```python
from build123d import *

# Parameters (mm, degrees)
SKETCH1_W      = 38.1
SKETCH1_H      = 38.1
BASEHEAD_DEPTH = 17.3736


with BuildPart() as part:
    # Sketch1 → BaseHead (new body)
    with BuildSketch(Plane(origin=(0, 0, 0), x_dir=(0, 0.7071067811865488, -0.7071067811865462), z_dir=(1, 0, 0))):
        Rectangle(SKETCH1_W, SKETCH1_H)
    extrude(amount=BASEHEAD_DEPTH)

    # BodySke → Body (revolve)
    with BuildSketch(Plane.XY, mode=Mode.PRIVATE) as body_sk:
        Polygon((17.3736, 0), (17.3736, 12.7), (91.6813, 12.7), (93.5736, 10.8077), (93.5736, 0), align=None)
    revolve(body_sk.sketch.rotate(Axis((0, 0, 0), (1, 0, 0)), 90), axis=Axis((0, 0, 0), (1, 0, 0)))

    # Sketch3 → HeadChamfer (revolve, cut)
    with BuildSketch(Plane.XY):
        Polygon((0, 19.05), (-12.7, 19.05), (-12.7, 52.340768363), (15.523740234, 52.340768363), align=None)
    revolve(axis=Axis((0, 0, 0), (1, 0, 0)), mode=Mode.SUBTRACT)


solid = part.part
```
Here's how the part is built. I have some questions about the finished solid (model axes, mm). A direction names the side the tool comes from. Give positions to 0.01 mm unless a question says otherwise; leave off trailing zeros. Loops run counter-clockwise (first coordinate to the right, second up) from the corner with the lowest first, then second, coordinate; pieces in that order, holes last. Notation, with made-up numbers: M -24.75,36.25 L 20.25,36.25 A24 cw 20.25,56.25 Z; hole C 14.25,-15.5 d11. An arc over 180 degrees is marked long. Put each result on its own line as item: value. Start each with the question number.
(1) I want a section at B-B on x = 30. Please give me the cut outline in (y, z), then the cut area to 3 significant figures.
(2) Will these pins go through, and if not, where does the flat tip stop? pin 1 Ø6 at (y, z) = (5.5, -13) entering from +X; pin 2 Ø1 at (y, z) = (3.5, 1) entering from -X; pin 3 Ø1 at (x, z) = (81.5, 11) entering from +Y; pin 4 Ø1.5 at (x, z) = (27.5, -6) entering from -Y.
(3) I want a section at A-A on x = 11.5. Please give me the cut outline in (y, z), then the cut area to 3 significant figures.
(4) If we mould it in two halves opening along X, with no side actions, what happens to faces 3 (the flat face through (0, 0, 0)), 4 (the flat face through (93.574, 0, 0)), 5 (the flat face through (8.57, -13.66, -13.28))? For each: +X half, -X half, draft (parallel to the pull), parting line (faces both ways), or undercut.
(5) I need wall thicknesses on line 1 along X through (y, z) = (-3, 18.5); line 2 along Y through (x, z) = (78, -8); line 3 along Z through (x, y) = (87, 7). Which ranges of each line are inside material? Lowest first, please. Write a range as [from, to].
(6) For faces 1 (the cylindrical face through (55, 7.7, -10.1)), 2 (the flat face through (8.57, -13.66, 13.28)), which set-ups out of +Z, -Z, +X, -X, +Y, -Y let a thin tool reach every point of the face, with its end or its side?
Answer block:
1. outline: C 0,0 d25.4
1. area: 507 mm^2
2. pin 1: x = 93.27
2. pin 2: x = 0
2. pin 3: y = 7.14
2. pin 4: y = -11.56
3. outline: M -26.94,0 L 0,-26.94 L 26.94,0 L 0,26.94 Z
3. area: 1,450 mm^2
4. face 3: -X half
4. face 4: +X half
4. face 5: draft
5. line 1: [0, 17.37]
5. line 2: [-9.86, 9.86]
5. line 3: [-10.6, 10.6]
6. face 1: +X
6. face 2: +Z, +X, -X, -Y
